Design review of the part built by this model. Coordinates are the model's own, in mm. Face numbers are marked on the shaded views. Coordinates: 2 decimals unless noted, no trailing zeros. Write each loop counter-clockwise with the first axis right and the second up, starting at its lowest first coordinate (ties: lowest second). Pieces come first, ordered by that corner, then holes.
Q1. For pin 1 Ø4 at (x, y) = (-45, -34) entering from -Z; pin 2 Ø1.5 at (y, z) = (36, 34.5) entering from +X; pin 3 Ø8 at (y, z) = (-36, 26.5) entering from +X, all flat-tipped, find the tip position at first contact; note any pin that passes through.
Q2. The part is to be moulded in two halves that separate along X. For the marked faces 1, 2 and 3, say which applies: released by +X, released by -X, zero draft, split by the parting line, or undercut.
Q3. Take a section at A-A, the plane y = 0. Write out the cut boundary in (x, z), plus the area to 3 significant figures.
Q4. For L1, parallel to X at y = 7.5, z = 30.5; L2, parallel to Y at x = 13.5, z = 10; L3, parallel to X at y = -12, z = 7, list the stretches that pass through material, from the lowest coordinate up.
Q5. Take a section at D-D, the plane z = 6. Write out the cut boundary in (x, y), plus the area to 3 significant figures.
Q6. Take a section at C-C, the plane z = 26.5. Write out the cut boundary in (x, y), plus the area to 3 significant figures.
from build123d import *

# Parameters (mm, degrees)
F2_R = 3


with BuildPart() as f1:
    # F0 (on Front) → F1 (revolve)
    with BuildSketch(Plane.XZ):
        with BuildLine():
            Line((-50, 0), (0, 0))
            Line((0, 0), (0, 1.5))
            Line((0, 1.5), (-34.5, 1.5))
            Line((-34.5, 1.5), (-35.5, 40))
            Line((-35.5, 40), (-50, 40))
            ThreePointArc((-50, 40), (-63.693287, 34.57717), (-69.960938, 21.249389))
            ThreePointArc((-69.960938, 21.249389), (-68.75, 20), (-69.960938, 18.750611))
            ThreePointArc((-69.960938, 18.750611), (-63.693287, 5.42283), (-50, 0))
        make_face()
    revolve(axis=Axis((0, 0, 20), (0, 0, 1)))

    # F2
    f2_edges = [f1.edges().sort_by_distance(p)[0] for p in [
        (35.5, 0, 40),
    ]]
    fillet(f2_edges, radius=F2_R)


solid = f1.part
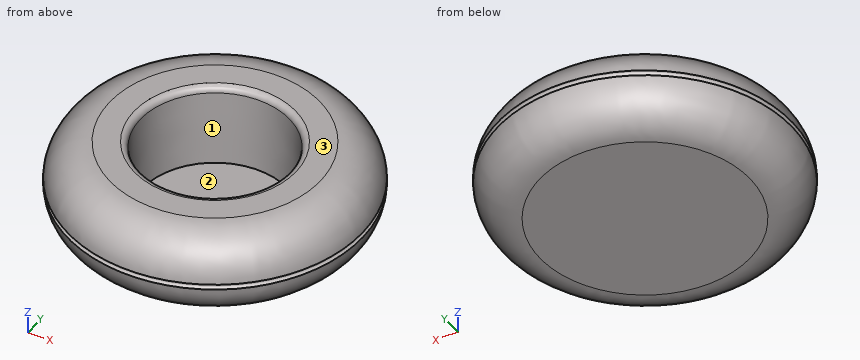
Responses:
1. pin 1: stops at z = 0.49
1. pin 2: stops at x = 53.68
1. pin 3: stops at x = 61.4
2. face 1: undercut
2. face 2: undercut
2. face 3: zero draft
3. outline: (-69.96, 18.75) arc R20 ccw to (-50, 0) - (50, 0) arc R20 ccw to (69.96, 18.75) arc R1.25 cw to (69.96, 21.25) arc R20 ccw to (50, 40) - (38.42, 40) arc R3 ccw to (35.42, 37.08) - (34.5, 1.5) - (-34.5, 1.5) - (-35.42, 37.08) arc R3 ccw to (-38.42, 40) - (-50, 40) arc R20 ccw to (-69.96, 21.25) arc R1.25 cw to start
3. area: 2,550 mm2
4. L1: x = -66.6 to -34.45, 34.45 to 66.6
4. L2: y = -65.95 to -31.99, 31.99 to 65.95
4. L3: x = -64.08 to -32.5, 32.5 to 64.08
5. outline: circle Ø128.57 at (0, 0); hole circle Ø69.23 at (0, 0)
5. area: 9,220 mm2
6. outline: circle Ø137.83 at (0, 0); hole circle Ø70.3 at (0, 0)
6. area: 11,000 mm2
